Verification items for the finished model (mm, model axes). Round coordinates to 2 decimals unless told otherwise and drop trailing zeros. Order: outer loops, then holes, each group sorted by start corner. A loop starts at its lowest first (then second) coordinate and runs counter-clockwise, first axis right, second up. Notation, with made-up numbers: (-32.75, 23.5) -> (-7.75, 23.5) arc R24 ccw to (-7.75, 36.5) -> close; hole circle Ø1 at (63.5, -5.75). An arc over 180 degrees is marked (long way). Put each result on its own line as item: value.
from build123d import *

# Parameters (mm, degrees)
SKETCH_1_W          = 20
SKETCH_1_H          = 20
EXTRUDE_1_DEPTH     = 2
SKETCH_2_R          = 1.5
CUT_EXTRUDE_1_DEPTH = 15.282856857
FILLET_1_R          = 3


with BuildPart() as part:
    # 草图1 → 凸台-拉伸1 (new body)
    with BuildSketch(Plane(origin=(0, 0, 0), x_dir=(1, 0, 0), z_dir=(0, 1, 0))):
        Rectangle(SKETCH_1_W, SKETCH_1_H)
    extrude(amount=EXTRUDE_1_DEPTH)

    # 草图2 → 切除-拉伸1 (cut, through all)
    with BuildSketch(Plane(origin=(0, 2, 0), x_dir=(1, 0, 0), z_dir=(0, 1, 0))):
        with Locations(Location((-5, 5, 0), (0, 0, 270))):
            Circle(SKETCH_2_R)
        with Locations(Location((5, 5, 0), (0, 0, 270))):
            Circle(SKETCH_2_R)
        with Locations(Location((-5, -5, 0), (0, 0, 270))):
            Circle(SKETCH_2_R)
        with Locations(Location((5, -5, 0), (0, 0, 270))):
            Circle(SKETCH_2_R)
    extrude(amount=-CUT_EXTRUDE_1_DEPTH, mode=Mode.SUBTRACT)

    # 圆角1
    fillet_1_edges = [part.edges().sort_by_distance(p)[0] for p in [
        (10, 1, 10),
        (-10, 1, 10),
        (-10, 1, -10),
        (10, 1, -10),
    ]]
    fillet(fillet_1_edges, radius=FILLET_1_R)


solid = part.part
Item 1: Section check D-D on z = 8. Record the boundary of the cut face in (x, y), then the cut area to 3 significant figures.
Check sheet entries:
outline: (-9.83, 0) -> (9.83, 0) -> (9.83, 2) -> (-9.83, 2) -> close
area: 39.3 mm^2
Item 2: Gauge pin test, flat ends, axial feed: pin 1 Ø4 at (x, z) = (5, 5) entering from +Y; pin 2 Ø2.5 at (x, z) = (-5, 5) entering from -Y. Record the tip position at first contact, or that the pin passes through.
Check sheet entries:
pin 1: stops at y = 2
pin 2: passes through
Item 3: Release check for a two-part mould opening along X. For faces 1 (the cylindrical face through (-3.99, 1.01, -6.11)), 2 (the cylindrical face through (-9.14, 1.01, -9.1)), 3 (the flat face through (0, 2, 0)), 4 (the cylindrical face through (5.07, 1.01, -6.5)) record: +X half, -X half, draft (parallel to the pull), parting line (faces both ways), or undercut.
Check sheet entries:
face 1: undercut
face 2: -X half
face 3: draft
face 4: undercut
Item 4: Section check C-C on y = 1.4. Record the boundary of the cut face in (x, z), then the cut area to 3 significant figures.
Check sheet entries:
outline: (-10, -7) arc R3 ccw to (-7, -10) -> (7, -10) arc R3 ccw to (10, -7) -> (10, 7) arc R3 ccw to (7, 10) -> (-7, 10) arc R3 ccw to (-10, 7) -> close; hole circle Ø3 at (-5, -5); hole circle Ø3 at (-5, 5); hole circle Ø3 at (5, -5); hole circle Ø3 at (5, 5)
area: 364 mm^2
Item 5: Section check B-B on x = 5. Record the boundary of the cut face in (y, z).
Check sheet entries:
outline: (0, -10) -> (2, -10) -> (2, -6.5) -> (0, -6.5) -> close; (0, -3.5) -> (2, -3.5) -> (2, 3.5) -> (0, 3.5) -> close; (0, 6.5) -> (2, 6.5) -> (2, 10) -> (0, 10) -> close
Item 6: Material ranges on L1, parallel to X at y = 0.75, z = -5; L2, parallel to X at y = 0.9, z = -4; L3, parallel to Z at x = -8.5, y = 0.25, recorded low to high. Write a range as [from, to].
Check sheet entries:
L1: x = [-10, -6.5], [-3.5, 3.5], [6.5, 10]
L2: x = [-10, -6.12], [-3.88, 3.88], [6.12, 10]
L3: z = [-9.6, 9.6]
Item 7: Section check A-A on z = -5. Record the boundary of the cut face in (x, y).
Check sheet entries:
outline: (-10, 0) -> (-6.5, 0) -> (-6.5, 2) -> (-10, 2) -> close; (-3.5, 0) -> (3.5, 0) -> (3.5, 2) -> (-3.5, 2) -> close; (6.5, 0) -> (10, 0) -> (10, 2) -> (6.5, 2) -> close
